Geometry: final body of the model. Coordinates: model frame, mm. Face numbers are marked on the shaded views. A direction names the side the tool comes from. Coordinates: 2 decimals unless noted, no trailing zeros. Write each loop counter-clockwise with the first axis right and the second up, starting at its lowest first coordinate (ties: lowest second). Pieces come first, ordered by that corner, then holes. Notation, with made-up numbers: (-10.75, 20.5) - (2.25, 20.5) arc R17 ccw to (2.25, 40.5) - close; hole circle Ø6 at (17, 31.5). An arc over 180 degrees is marked (long way). Answer as a JSON object with one key per item and string values. Group by question number.
Item 1: Section B-B on x = -15. Return loops of the section in (y, z), and give its area (3 significant figures).
Item 2: Mould query, pull axis Z, two halves, no side actions, for the marked faces 4, 5 and 6. Classes: pulls with the +Z half, pulls with the -Z half, needs draft (parallel to the pull), parting line crosses it, or undercut.
Item 3: First-contact query: pin 1 Ø9 at (x, y) = (-2.5, -33) entering from +Z; pin 2 Ø5 at (x, y) = (-28, 20) entering from -Z; pin 3 Ø1.5 at (x, y) = (29, -26) entering from +Z; pin 4 Ø0.6 at (y, z) = (2, 2.5) entering from -X. Flat tips, straight axial feed; report the tip coordinate or a pass-through.
Item 4: Section C-C on z = 13.75. State how many separate pieces and enclosed holes the cut face has, and give its area (3 significant figures).
Item 5: Section D-D on x = -23. Return loops of the section in (y, z).
Item 6: Line query: line 1 along X through (y, z) = (-28, 19.8); line 2 along X through (y, z) = (-21, 4.5); line 3 along X through (y, z) = (11, 14.75). Output: solid intervals per line, ascending. Write a range as from..to.
Item 7: Set-up query: the marked faces 1, 2 and 3. Return all of +Z, -Z, +X, -X, +Y, -Y with unobstructed straight access to the full face (end or side cutting, diameter ignored); none if empty.
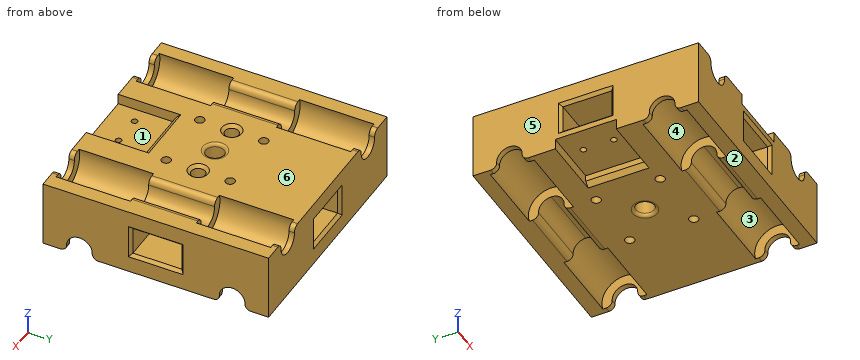
```python
from build123d import *

# Parameters (mm, degrees)
SKETCH018_R          = 5
SKETCH018_R_2        = 1.525
PAD005_DEPTH         = 6.4
SKETCH019_R          = 5
SKETCH019_R_2        = 1.525
SKETCH019_R_3        = 2.25
PAD006_DEPTH         = 6.4
CHAMFER004_SIZE      = 1
SKETCH020_R          = 5
SKETCH020_R_2        = 3
PAD007_DEPTH         = 22
FILLET005_R          = 1
SKETCH015_W          = 74
SKETCH015_H          = 74
PAD004_DEPTH         = 22
SKETCH016_W          = 16
SKETCH016_H          = 9.2
POCKET010_DEPTH      = 37.001
POCKET010_DEPTH_BACK = -37.001
SKETCH017_W          = 16
SKETCH017_H          = 9.2
POCKET011_DEPTH      = 37.001
POCKET011_DEPTH_BACK = -37.001
FILLET004_R          = 2
CHAMFER003_SIZE      = 1
SKETCH021_W          = 20
SKETCH021_H          = 19
POCKET012_DEPTH      = 3.5
SKETCH022_W          = 19
SKETCH022_H          = 20
POCKET013_DEPTH      = 3.5
SKETCH023_R          = 1
POCKET014_DEPTH      = 2.9
SKETCH024_R          = 1
POCKET015_DEPTH      = 2.9
FILLET006_R          = 2
CHAMFER_SIZE         = 1.5


with BuildPart() as body006:
    # Sketch026 → Revolution001 (revolve)
    with BuildSketch(Plane.YZ):
        Polygon((-37, 4.2), (-37, 0), (37, 0), (37, 4.2), (35.2, 4.2), (35.2, 7.55), (10.8, 7.55), (10.8, 4.2), (-10.8, 4.2), (-10.8, 7.55), (-35.2, 7.55), (-35.2, 4.2), align=None)
    revolve(axis=Axis((0, 0, 0), (0, 1, 0)))


with BuildPart() as body006_1:
    # Body006 placement: moved
    add(body006.part.moved(Location((-25.05, 0, 19.8))))


with BuildPart() as body007:
    # Sketch027 → Revolution002 (revolve)
    with BuildSketch(Plane.XZ):
        Polygon((-37, 4.2), (-37, 0), (37, 0), (37, 4.2), (35.2, 4.2), (35.2, 7.55), (10.8, 7.55), (10.8, 4.2), (-10.8, 4.2), (-10.8, 7.55), (-35.2, 7.55), (-35.2, 4.2), align=None)
    revolve(axis=Axis((0, 0, 0), (1, 0, 0)))


with BuildPart() as body007_1:
    # Body007 placement: moved
    add(body007.part.moved(Location((0, 25.05, 2.2))))


with BuildPart() as body008:
    # Sketch028 → Revolution003 (revolve)
    with BuildSketch(Plane.XZ):
        Polygon((-37, 4.2), (-37, 0), (37, 0), (37, 4.2), (35.2, 4.2), (35.2, 7.55), (10.8, 7.55), (10.8, 4.2), (-10.8, 4.2), (-10.8, 7.55), (-35.2, 7.55), (-35.2, 4.2), align=None)
    revolve(axis=Axis((0, 0, 0), (1, 0, 0)))


with BuildPart() as body008_1:
    # Body008 placement: moved
    add(body008.part.moved(Location((0, -25.05, 2.2))))


with BuildPart() as bearingholes:
    # Sketch025 → Revolution (revolve)
    with BuildSketch(Plane.YZ):
        Polygon((-37, 4.2), (-37, 0), (37, 0), (37, 4.2), (35.2, 4.2), (35.2, 7.55), (10.8, 7.55), (10.8, 4.2), (-10.8, 4.2), (-10.8, 7.55), (-35.2, 7.55), (-35.2, 4.2), align=None)
    revolve(axis=Axis((0, 0, 0), (0, 1, 0)))


with BuildPart() as bearingholes_1:
    # Body005 placement: moved
    add(bearingholes.part.moved(Location((25.05, 0, 19.8))))

    # Fusion001: union Body006, Body007, Body008
    add(body006_1.part)
    add(body007_1.part)
    add(body008_1.part)


with BuildPart() as innercorebottom:
    # Sketch018 → Pad005 (new body)
    with BuildSketch(Plane.XY):
        with BuildLine():
            Line((-16, 18), (16, 18))
            ThreePointArc((18, 16), (17.414214, 17.414214), (16, 18))
            Line((18, 16), (18, -16))
            ThreePointArc((16, -18), (17.414214, -17.414214), (18, -16))
            Line((16, -18), (-16, -18))
            ThreePointArc((-18, -16), (-17.414214, -17.414214), (-16, -18))
            Line((-18, -16), (-18, 16))
            ThreePointArc((-16, 18), (-17.414214, 17.414214), (-18, 16))
        make_face()
        Circle(SKETCH018_R, mode=Mode.SUBTRACT)
        with Locations((-10.5, 10.5)):
            Circle(SKETCH018_R_2, mode=Mode.SUBTRACT)
        with Locations((10.5, 10.5)):
            Circle(SKETCH018_R_2, mode=Mode.SUBTRACT)
        with Locations((10.5, -10.5)):
            Circle(SKETCH018_R_2, mode=Mode.SUBTRACT)
        with Locations((-10.5, -10.5)):
            Circle(SKETCH018_R_2, mode=Mode.SUBTRACT)
    extrude(amount=PAD005_DEPTH)


with BuildPart() as innercoretop:
    # Sketch019 → Pad006 (new body)
    with BuildSketch(Plane.XY):
        with BuildLine():
            Line((-16, 18), (16, 18))
            ThreePointArc((18, 16), (17.414214, 17.414214), (16, 18))
            Line((18, 16), (18, -16))
            ThreePointArc((16, -18), (17.414214, -17.414214), (18, -16))
            Line((16, -18), (-16, -18))
            ThreePointArc((-18, -16), (-17.414214, -17.414214), (-16, -18))
            Line((-18, -16), (-18, 16))
            ThreePointArc((-16, 18), (-17.414214, 17.414214), (-18, 16))
        make_face()
        Circle(SKETCH019_R, mode=Mode.SUBTRACT)
        with Locations((-10.5, 10.5)):
            Circle(SKETCH019_R_2, mode=Mode.SUBTRACT)
        with Locations((10.5, 10.5)):
            Circle(SKETCH019_R_2, mode=Mode.SUBTRACT)
        with Locations((10.5, -10.5)):
            Circle(SKETCH019_R_2, mode=Mode.SUBTRACT)
        with Locations((-10.5, -10.5)):
            Circle(SKETCH019_R_2, mode=Mode.SUBTRACT)
        with Locations((-10.5, 0)):
            Circle(SKETCH019_R_3, mode=Mode.SUBTRACT)
        with Locations((10.5, 0)):
            Circle(SKETCH019_R_3, mode=Mode.SUBTRACT)
    extrude(amount=-PAD006_DEPTH)

    # Chamfer004
    chamfer004_edges = [innercoretop.edges().sort_by_distance(p)[0] for p in [
        (-12.75, 0, 0),
        (8.25, 0, 0),
    ]]
    chamfer(chamfer004_edges, length=CHAMFER004_SIZE)


with BuildPart() as innercoretop_1:
    # Body003 placement: moved
    add(innercoretop.part.moved(Location((0, 0, 22))))


with BuildPart() as centerhole:
    # Sketch020 → Pad007 (new body)
    with BuildSketch(Plane.XY):
        Circle(SKETCH020_R)
        Circle(SKETCH020_R_2, mode=Mode.SUBTRACT)
    extrude(amount=PAD007_DEPTH)

    # Fillet005
    fillet005_edges = [centerhole.edges().sort_by_distance(p)[0] for p in [
        (-3, 0, 22),
        (-3, 0, 0),
    ]]
    fillet(fillet005_edges, radius=FILLET005_R)


with BuildPart() as chamfer_body:
    # Sketch015 → Pad004 (new body)
    with BuildSketch(Plane.XY):
        Rectangle(SKETCH015_W, SKETCH015_H)
        with BuildLine():
            Line((-16, 18), (16, 18))
            ThreePointArc((18, 16), (17.414214, 17.414214), (16, 18))
            Line((18, 16), (18, -16))
            ThreePointArc((16, -18), (17.414214, -17.414214), (18, -16))
            Line((16, -18), (-16, -18))
            ThreePointArc((-18, -16), (-17.414214, -17.414214), (-16, -18))
            Line((-18, -16), (-18, 16))
            ThreePointArc((-16, 18), (-17.414214, 17.414214), (-18, 16))
        make_face(mode=Mode.SUBTRACT)
    extrude(amount=PAD004_DEPTH)

    # Sketch016 → Pocket010 (cut, two sides)
    with BuildSketch(Plane.YZ) as pocket010_sk:
        with Locations((0, 11)):
            Rectangle(SKETCH016_W, SKETCH016_H)
    extrude(amount=-POCKET010_DEPTH, mode=Mode.SUBTRACT)
    extrude(pocket010_sk.sketch, amount=-POCKET010_DEPTH_BACK, mode=Mode.SUBTRACT)

    # Sketch017 → Pocket011 (cut, two sides)
    with BuildSketch(Plane.XZ) as pocket011_sk:
        with Locations((0, 11)):
            Rectangle(SKETCH017_W, SKETCH017_H)
    extrude(amount=-POCKET011_DEPTH, mode=Mode.SUBTRACT)
    extrude(pocket011_sk.sketch, amount=-POCKET011_DEPTH_BACK, mode=Mode.SUBTRACT)

    # Fillet004
    fillet004_edges = [chamfer_body.edges().sort_by_distance(p)[0] for p in [
        (-18, -8, 11),
        (-18, 8, 11),
        (-8, -18, 11),
        (8, -18, 11),
        (-8, 18, 11),
        (8, 18, 11),
        (18, 8, 11),
        (18, -8, 11),
    ]]
    fillet(fillet004_edges, radius=FILLET004_R)

    # Chamfer003
    chamfer003_edges = [chamfer_body.edges().sort_by_distance(p)[0] for p in [
        (0, 37, 15.6),
        (8, 37, 11),
        (0, 37, 6.4),
        (-8, 37, 11),
        (-37, 8, 11),
        (-37, 0, 15.6),
        (-37, -8, 11),
        (-37, 0, 6.4),
        (-8, -37, 11),
        (0, -37, 15.6),
        (0, -37, 6.4),
        (8, -37, 11),
        (37, 8, 11),
        (37, 0, 15.6),
        (37, 0, 6.4),
        (37, -8, 11),
    ]]
    chamfer(chamfer003_edges, length=CHAMFER003_SIZE)

    # Sketch021 (on Face15 of Chamfer003) → Pocket012 (cut)
    with BuildSketch(Plane.XY.offset(22)):
        with Locations((0, -27.5)):
            Rectangle(SKETCH021_W, SKETCH021_H)
    extrude(amount=-POCKET012_DEPTH, mode=Mode.SUBTRACT)

    # Sketch022 (on Face14 of Pocket012) → Pocket013 (cut)
    with BuildSketch(Plane(origin=(0, 0, 0), x_dir=(1, 0, 0), z_dir=(0, 0, -1))):
        with Locations((-27.5, 0)):
            Rectangle(SKETCH022_W, SKETCH022_H)
    extrude(amount=-POCKET013_DEPTH, mode=Mode.SUBTRACT)

    # Sketch023 (on Face46 of Pocket013) → Pocket014 (cut)
    with BuildSketch(Plane.XY.offset(18.5)):
        with Locations((-5, -29)):
            Circle(SKETCH023_R)
        with Locations((5, -29)):
            Circle(SKETCH023_R)
    extrude(amount=-POCKET014_DEPTH, mode=Mode.SUBTRACT)

    # Sketch024 (on Face29 of Pocket014) → Pocket015 (cut)
    with BuildSketch(Plane(origin=(0, 0, 3.5), x_dir=(1, 0, 0), z_dir=(0, 0, -1))):
        with Locations((-29, 5)):
            Circle(SKETCH024_R)
        with Locations((-29, -5)):
            Circle(SKETCH024_R)
    extrude(amount=-POCKET015_DEPTH, mode=Mode.SUBTRACT)

    # Fusion: union InnerCoreBottom, InnerCoreTop, CenterHole
    add(innercorebottom.part)
    add(innercoretop_1.part)
    add(centerhole.part)

    # Cut: cut BearingHoles
    add(bearingholes_1.part, mode=Mode.SUBTRACT)

    # Fillet006
    fillet006_edges = [chamfer_body.edges().sort_by_distance(p)[0] for p in [
        (-36.1, 28.627709, 0),
        (0, 28.627709, 0),
        (36.1, 28.627709, 0),
        (28.627709, 36.1, 22),
        (28.627709, 0, 22),
        (28.627709, -36.1, 22),
        (21.472291, 36.1, 22),
        (-21.472291, 36.1, 22),
        (-28.627709, 36.1, 22),
        (-28.627709, -36.1, 22),
        (-28.627709, 0, 22),
        (36.1, 21.472291, 0),
        (36.1, -21.472291, 0),
        (36.1, -28.627709, 0),
        (0, -28.627709, 0),
        (-36.1, -28.627709, 0),
        (21.472291, 0, 22),
        (21.472291, -36.1, 22),
        (-21.472291, -36.1, 22),
        (-21.472291, 0, 22),
        (-36.1, -21.472291, 0),
        (-36.1, 21.472291, 0),
        (0, -21.472291, 0),
        (0, 21.472291, 0),
    ]]
    fillet(fillet006_edges, radius=FILLET006_R)

    # Chamfer
    chamfer_edges = [chamfer_body.edges().sort_by_distance(p)[0] for p in [
        (0, -18, 22),
        (-18, 0, 0),
    ]]
    chamfer(chamfer_edges, length=CHAMFER_SIZE)


solid = chamfer_body.part
```
Checks:
{
 "1": {"outline": "(-37, 0) - (-32.27, 0) arc R7.55 cw (long way) to (-17.83, 0) - (17.83, 0) arc R7.55 cw (long way) to (32.27, 0) - (37, 0) - (37, 22) - (-37, 22) - close; hole (-18, 6.4) - (18, 6.4) - (18, 15.6) - (-18, 15.6) - close", "area": "1,050 mm^2"},
 "2": {"face 4": "undercut", "face 5": "needs draft", "face 6": "pulls with the +Z half"},
 "3": {"pin 1": "z = 18.5", "pin 2": "z = 0", "pin 3": "z = 13.89", "pin 4": "x = -18"},
 "4": {"separate pieces": "5", "enclosed holes": "5", "area": "2,130 mm^2"},
 "5": {"outline": "(-37, 0) - (-32.27, 0) arc R7.55 cw (long way) to (-17.83, 0) - (-10, 0) - (-10, 3.5) - (10, 3.5) - (10, 0) - (17.83, 0) arc R7.55 cw (long way) to (32.27, 0) - (37, 0) - (37, 16.13) - (35.2, 16.13) - (35.2, 12.53) - (10.8, 12.53) - (10.8, 16.13) - (-10.8, 16.13) - (-10.8, 12.53) - (-35.2, 12.53) - (-35.2, 16.13) - (-37, 16.13) - close; hole (-8, 6.4) - (8, 6.4) - (8, 15.6) - (-8, 15.6) - close"},
 "6": {"line 1": "-37..-32.6, -17.5..-10, 10..17.5, 32.6..37", "line 2": "-37..-35.2, -10.8..10.8, 35.2..37", "line 3": "-37..-30.66, -19.44..-18, 18..19.44, 30.66..37"},
 "7": {"face 1": "+Z, -Y", "face 2": "-Z, +X, -X, +Y, -Y", "face 3": "none"}
}
